```python
from build123d import *

# Parameters (mm, degrees)
SALIENTE_EXTRUIR1_DEPTH = 19
CORTAR_EXTRUIR1_REACH   = 84.816
CROQUIS2_R              = 5
CORTAR_EXTRUIR2_REACH   = 84.816
CROQUIS3_R              = 5
SALIENTE_EXTRUIR2_DEPTH = 12
CROQUIS5_R              = 3.5
SALIENTE_EXTRUIR3_DEPTH = 20
SALIENTE_EXTRUIR4_DEPTH = 13.3
REDONDEO1_R             = 1.5
CROQUIS8_R              = 2.5
SALIENTE_EXTRUIR5_DEPTH = 1.85
REDONDEO2_R             = 1.5
SIMETR_A1_START         = -1.3500001
SIMETR_A1_OUTLINE_R     = 2.5
SIMETR_A1_DEPTH         = 1.3500001
SIMETR_A1_START_2       = -13.3
SIMETR_A1_2_DEPTH       = 26.6
SIMETR_A1_START_3       = -3
SIMETR_A1_5_DEPTH       = 3


with BuildPart() as part:
    # Croquis1 → Saliente-Extruir1 (new body)
    with BuildSketch(Plane(origin=(0, 0, 0), x_dir=(1, 0, 0), z_dir=(0, 1, 0))):
        with BuildLine():
            Line((-25.4, 23.25), (-25.4, 38.25))
            Line((-25.4, 38.25), (25.4, 38.25))
            Line((25.4, 38.25), (25.4, -13.25))
            Line((25.4, -13.25), (-5.6, -13.25))
            ThreePointArc((-5.6, -13.25), (-10.6, -18.25), (-5.6, -23.25))
            Line((-5.6, -23.25), (25.4, -23.25))
            Line((25.4, -23.25), (25.4, -38.25))
            Line((25.4, -38.25), (-25.4, -38.25))
            Line((-25.4, -38.25), (-25.4, 13.25))
            Line((-25.4, 13.25), (5.6, 13.25))
            ThreePointArc((5.6, 13.25), (10.6, 18.25), (5.6, 23.25))
            Line((5.6, 23.25), (-25.4, 23.25))
        make_face()
    extrude(amount=SALIENTE_EXTRUIR1_DEPTH)

    # Croquis2 → Cortar-Extruir1 (cut, up to next)
    with BuildSketch(Plane(origin=(0, 0, -38.25), x_dir=(-1, 0, 0), z_dir=(0, 0, -1)), mode=Mode.PRIVATE) as cortar_extruir1_sk1:
        with Locations((0, 9.5)):
            Circle(CROQUIS2_R)
    cortar_extruir1_tool1 = extrude(cortar_extruir1_sk1.sketch, amount=-CORTAR_EXTRUIR1_REACH, mode=Mode.PRIVATE) & part.part
    add(cortar_extruir1_tool1.solids().sort_by_distance((0, 9.5, -38.25))[0], mode=Mode.SUBTRACT)

    # Croquis3 → Cortar-Extruir2 (cut, up to next)
    with BuildSketch(Plane.XY.offset(38.25), mode=Mode.PRIVATE) as cortar_extruir2_sk1:
        with Locations(Location((0, 9.5, 0), (0, 0, 180))):
            Circle(CROQUIS3_R)
    cortar_extruir2_tool1 = extrude(cortar_extruir2_sk1.sketch, amount=-CORTAR_EXTRUIR2_REACH, mode=Mode.PRIVATE) & part.part
    add(cortar_extruir2_tool1.solids().sort_by_distance((0, 9.5, 38.25))[0], mode=Mode.SUBTRACT)

    # Croquis4 → Saliente-Extruir2 (add)
    with BuildSketch(Plane(origin=(25.4, 0, 0), x_dir=(0, 0, -1), z_dir=(1, 0, 0))):
        Polygon((0.567837029, 2.595106003), (6.263732126, 6.539314294), (5.695895097, 13.444208291), (-0.567837029, 16.404893997), (-6.263732126, 12.460685706), (-5.695895097, 5.555791709), align=None)
    extrude(amount=SALIENTE_EXTRUIR2_DEPTH)

    # Croquis5 → Saliente-Extruir3 (add)
    with BuildSketch(Plane(origin=(37.4, 0, 0), x_dir=(0, 0, -1), z_dir=(1, 0, 0))):
        with Locations((0, 9.5)):
            Circle(CROQUIS5_R)
    extrude(amount=SALIENTE_EXTRUIR3_DEPTH)

    # Croquis6 → Saliente-Extruir4 (add, symmetric)
    with BuildSketch(Plane.XY):
        with BuildLine():
            Line((25.4, 19), (15.884301947, 19))
            ThreePointArc((15.884301947, 19), (15.401815848, 19.020910233), (14.922947827, 19.08348413))
            Line((14.922947827, 19.08348413), (11.877052173, 19.61651587))
            ThreePointArc((11.877052173, 19.61651587), (11.398184152, 19.679089767), (10.915698053, 19.7))
            Line((10.915698053, 19.7), (-25.4, 19.7))
            Line((-25.4, 19.7), (-25.4, 20.7))
            Line((-25.4, 20.7), (10.915698053, 20.7))
            ThreePointArc((10.915698053, 20.7), (11.398184152, 20.679089767), (11.877052173, 20.61651587))
            Line((11.877052173, 20.61651587), (14.922947827, 20.08348413))
            ThreePointArc((14.922947827, 20.08348413), (15.401815848, 20.020910233), (15.884301947, 20))
            Line((15.884301947, 20), (25.4, 20))
            Line((25.4, 20), (25.4, 19))
        make_face()
    extrude(amount=SALIENTE_EXTRUIR4_DEPTH, both=True)

    # Redondeo1
    redondeo1_edges = [part.edges().sort_by_distance(p)[0] for p in [
        (-25.4, 20.2, -13.3),
        (-25.4, 20.2, 13.3),
        (25.4, 19.5, 13.3),
        (25.4, 19.5, -13.3),
    ]]
    fillet(redondeo1_edges, radius=REDONDEO1_R)

    # Croquis8 → Saliente-Extruir5 (add)
    with BuildSketch(Plane(origin=(0, 20, 0), x_dir=(1, 0, 0), z_dir=(0, 1, 0))):
        with Locations(Location((19.892150974, 9.3, 0), (0, 0, 180))):
            Circle(CROQUIS8_R)
        with Locations(Location((19.892150974, -9.3, 0), (0, 0, 180))):
            Circle(CROQUIS8_R)
    extrude(amount=SALIENTE_EXTRUIR5_DEPTH)

    # Redondeo2
    redondeo2_edges = [part.edges().sort_by_distance(p)[0] for p in [
        (22.392150974, 21.85, -9.3),
        (22.392150974, 21.85, 9.3),
    ]]
    fillet(redondeo2_edges, radius=REDONDEO2_R)

    # Simetría1: read off the stored shape, not the designer's step
    # Simetría1 outline → Simetría1 (add)
    with BuildSketch(Plane(origin=(0, 0, 0), x_dir=(1, 0, 0), z_dir=(0, 1, 0)).offset(SIMETR_A1_START)):
        with Locations((19.892150974, 9.3)):
            Circle(SIMETR_A1_OUTLINE_R)
        with Locations((19.892150974, -9.3)):
            Circle(SIMETR_A1_OUTLINE_R)
    extrude(amount=SIMETR_A1_DEPTH)

    # Simetr_a1 2 outline → Simetr_a1 2 (add)
    with BuildSketch(Plane.XY.offset(SIMETR_A1_START_2)):
        with BuildLine():
            Line((-25.4, -0.7), (-25.4, -1.7))
            Line((-25.4, -1.7), (10.915698053, -1.7))
            ThreePointArc((10.915698053, -1.7), (11.398184152, -1.679089767), (11.877052173, -1.61651587))
            Line((11.877052173, -1.61651587), (14.922947827, -1.08348413))
            ThreePointArc((14.922947827, -1.08348413), (15.401815848, -1.020910233), (15.884301947, -1))
            Line((15.884301947, -1), (25.4, -1))
            Line((25.4, -1), (25.4, 0))
            Line((25.4, 0), (15.884301947, 0))
            ThreePointArc((15.884301947, 0), (15.401815848, -0.020910233), (14.922947827, -0.08348413))
            Line((14.922947827, -0.08348413), (11.877052173, -0.61651587))
            ThreePointArc((11.877052173, -0.61651587), (11.398184152, -0.679089767), (10.915698053, -0.7))
            Line((10.915698053, -0.7), (-25.4, -0.7))
        make_face()
    extrude(amount=SIMETR_A1_2_DEPTH)

    # Simetr_a1 3 outline → Simetr_a1 3 (revolve)
    with BuildSketch(Plane(origin=(19.892150974, 0, -9.3), x_dir=(1, 0, 0), z_dir=(0, 0, 1))):
        with BuildLine():
            Line((0, -1.35), (0, -2.85))
            Line((0, -2.85), (1, -2.85))
            ThreePointArc((1, -2.85), (2.060660172, -2.410660172), (2.5, -1.35))
            Line((2.5, -1.35), (0, -1.35))
        make_face()
    revolve(axis=Axis((19.892150974, 0, -9.3), (0, 1, 0)))

    # Simetr_a1 4 outline → Simetr_a1 4 (revolve)
    with BuildSketch(Plane(origin=(19.892150974, 0, 9.3), x_dir=(1, 0, 0), z_dir=(0, 0, 1))):
        with BuildLine():
            Line((0, -1.35), (0, -2.85))
            Line((0, -2.85), (1, -2.85))
            ThreePointArc((1, -2.85), (2.060660172, -2.410660172), (2.5, -1.35))
            Line((2.5, -1.35), (0, -1.35))
        make_face()
    revolve(axis=Axis((19.892150974, 0, 9.3), (0, 1, 0)))

    # Simetr_a1 5 outline → Simetr_a1 5 (cut)
    with BuildSketch(Plane(origin=(0, 0, 0), x_dir=(1, 0, 0), z_dir=(0, 1, 0)).offset(SIMETR_A1_START_3)):
        with BuildLine():
            ThreePointArc((-25.4, 11.8), (-24.960660172, 12.860660172), (-23.9, 13.3))
            Line((-23.9, 13.3), (-25.4, 13.3))
            Line((-25.4, 13.3), (-25.4, 11.8))
        make_face()
        with BuildLine():
            Line((25.4, 13.3), (23.9, 13.3))
            ThreePointArc((23.9, 13.3), (24.960660172, 12.860660172), (25.4, 11.8))
            Line((25.4, 11.8), (25.4, 13.3))
        make_face()
        with BuildLine():
            ThreePointArc((-23.9, -13.3), (-24.960660172, -12.860660172), (-25.4, -11.8))
            Line((-25.4, -11.8), (-25.4, -13.3))
            Line((-25.4, -13.3), (-23.9, -13.3))
        make_face()
        with BuildLine():
            Line((25.4, -13.3), (25.4, -11.8))
            ThreePointArc((25.4, -11.8), (24.960660172, -12.860660172), (23.9, -13.3))
            Line((23.9, -13.3), (25.4, -13.3))
        make_face()
    extrude(amount=SIMETR_A1_5_DEPTH, mode=Mode.SUBTRACT)


solid = part.part
```
CAD build for the part. Positions are in the model's coordinates, mm. A direction names the side the tool comes from. Round coordinates to 2 decimals unless told otherwise and drop trailing zeros. Write each loop counter-clockwise with the first axis right and the second up, starting at its lowest first coordinate (ties: lowest second). Pieces come first, ordered by that corner, then holes. Notation, with made-up numbers: (74, 28.5) - (106, 28.5) arc R16 ccw to (106, 36.5) - close; hole circle Ø6 at (26.5, 25.25). An arc over 180 degrees is marked (long way). Write item = value, one per line. Start each with the question number.
Q1. Probe L1, parallel to Y at x = -6, z = 10.5; L2, parallel to Z at x = 3.5, y = 4.5; L3, parallel to X at y = 9.5, z = 35. List the from-to ranges inside material, lowest first. Write a range as from..to.
Q2. Band-saw the part on C-C (y = 9.5). Count the separate pieces of the cut face and the enclosed holes in it, then the cut area to 3 significant figures.
Q3. Band-saw the part on A-A (x = 0). Give the cut face in (y, z), then the cut area to 3 significant figures.
Q4. Band-saw the part on D-D (z = 29.5). Give the cut face in (x, y).
Q5. Mould opens along Y. For faces 1 (the flat face through (31.316, 14.904, -2.608)), 2 (the cylindrical face through (0.651, 14.457, -30.855)), 3 (the flat face through (13.421, -0.346, -0.186)) say: pulls with the +Y half, pulls with the -Y half, needs draft (parallel to the pull), parting line crosses it, or undercut.
Q6. Which spindle directions (+Z, -Z, +X, -X, +Y, -Y) get a long thin tool onto all of the face, cutting with end or side? Do faces 4 (the flat face through (13.379, 20.354, 0.186)), 5 (the flat face through (-7, 20.7, 0)), 6 (the flat face through (31.316, 9.943, -5.984)). Say none if no direction does.
Q7. Band-saw the part on B-B (x = -12.5). Give the cut face in (y, z), then the cut area to 3 significant figures.
Q8. Drop flat-ended pins along their axis: pin 1 (1.4 mm diameter, centred on x = 6.5, y = 20, fed in from +Z); pin 2 (10 mm diameter, centred on x = 9, z = -16.5, fed in from +Y); pin 3 (2 mm diameter, centred on x = 42, y = 7, fed in from +Z). Give the stop position or say it passes through.
Answers below:
q1.L1 = -1.7..-0.7, 0..19, 19.7..20.7
q1.L2 = -38.25..-23.25, -13.25..13.25, 23.25..38.25
q1.L3 = -25.4..-5, 5..25.4
q2.separate_pieces = 3
q2.enclosed_holes = 0
q2.area = 3,170 mm2
q3.outline = (-1.7, -13.3) - (-0.7, -13.3) - (-0.7, 13.3) - (-1.7, 13.3) - close; (0, -38.25) - (4.5, -38.25) - (4.5, -23.25) - (0, -23.25) - close; (0, -13.25) - (19, -13.25) - (19, 13.25) - (0, 13.25) - close; (0, 23.25) - (4.5, 23.25) - (4.5, 38.25) - (0, 38.25) - close; (14.5, -38.25) - (19, -38.25) - (19, -23.25) - (14.5, -23.25) - close; (14.5, 23.25) - (19, 23.25) - (19, 38.25) - (14.5, 38.25) - close; (19.7, -13.3) - (20.7, -13.3) - (20.7, 13.3) - (19.7, 13.3) - close
q3.area = 827 mm2
q4.outline = (-25.4, 0) - (25.4, 0) - (25.4, 19) - (-25.4, 19) - close; hole circle Ø10 at (0, 9.5)
q5.face_1 = pulls with the +Y half
q5.face_2 = undercut
q5.face_3 = undercut
q6.face_4 = +Z, -Z, +Y
q6.face_5 = +Z, -Z, -X, +Y
q6.face_6 = -Z, +X, +Y
q7.outline = (-1.7, -13.3) - (-0.7, -13.3) - (-0.7, 13.3) - (-1.7, 13.3) - close; (0, -38.25) - (19, -38.25) - (19, -23.25) - (0, -23.25) - close; (0, -13.25) - (19, -13.25) - (19, 38.25) - (0, 38.25) - close; (19.7, -13.3) - (20.7, -13.3) - (20.7, 13.3) - (19.7, 13.3) - close
q7.area = 1,320 mm2
q8.pin_1 = 13.3
q8.pin_2 = 20.7
q8.pin_3 = 3.16
